Verification items for the finished model (mm, model axes). A direction names the side the tool comes from. Coordinates: 2 decimals unless noted, no trailing zeros. Order: outer loops, then holes, each group sorted by start corner. A loop starts at its lowest first (then second) coordinate and runs counter-clockwise, first axis right, second up. Notation, with made-up numbers: (82, -25) -> (97, -25) arc R24 cw to (97, 5) -> close; hole circle Ø6 at (13, 40.25). An arc over 180 degrees is marked (long way). Answer as CSV lines item,"result".
```python
from build123d import *

# Parameters (mm, degrees)
F0_W        = 10.5280357461
F0_H        = 21.2543252856
F1_DEPTH    = 30
F2_R        = 5
F3_R        = 2
F4_R        = 2
F5_R        = 2
F6_R        = 7
F7_T1_DEPTH = 81.4336597593
F8_R        = 10
F9_R        = 1
F10_R       = 10
F11_R       = 10
F13_DEPTH   = 30
F14_R       = 2


# Not quite as in the source:
# - a fillet or chamfer that OpenCascade refuses, or shapes differently, is made with other operations: its cross-section is extruded or revolved along the edge and cut away or added


with BuildPart() as f1:
    # F0 (on Top) → F1 (new body)
    with BuildSketch(Plane.XY):
        Polygon((23.4277165425, 17.0276444405), (-54.4175144403, 17.0276444405), (-54.4175144403, 8.6288927123), (12.8996807964, 8.6288927123), (23.4277165425, 8.6288927123), align=None)
        with Locations((18.1636986695, -1.9982699305)):
            Rectangle(F0_W, F0_H)
        Polygon((23.4277165425, -21.8901360014), (23.4277165425, -12.6254325733), (12.8996807964, -12.6254325733), (-40.6902853517, -12.6254325733), (-40.6902853517, -21.8901360014), (-27.7488247443, -21.8901360014), (-19.1767220313, -21.8901360014), align=None)
        with BuildLine():
            Line((-19.1767220313, -43.3673763092), (-19.1767220313, -21.8901360014))
            Line((-19.1767220313, -21.8901360014), (-27.7488247443, -21.8901360014))
            ThreePointArc((-27.7488247443, -21.8901360014), (-24.844212154, -33.1801228498), (-19.1767220313, -43.3673763092))
        make_face()
        with BuildLine():
            Line((-27.7488247443, -21.8901360014), (-40.6902853517, -21.8901360014))
            ThreePointArc((-40.6902853517, -21.8901360014), (-35.4626283769, -44.0139601174), (-20.8854291365, -61.4580781309))
            ThreePointArc((-20.8854291365, -61.4580781309), (-15.0806794225, -65.2011539101), (-8.8108392586, -68.098538912))
            ThreePointArc((-8.8108392586, -68.098538912), (11.6035028188, -71.235670703), (31.5175838768, -65.7569542527))
            Line((31.5175838768, -65.7569542527), (34.4113459094, -58.7176481952))
            ThreePointArc((34.4113459094, -58.7176481952), (5.0047282318, -60.1630877212), (-19.1767220313, -43.3673763092))
            ThreePointArc((-19.1767220313, -43.3673763092), (-24.844212154, -33.1801228498), (-27.7488247443, -21.8901360014))
        make_face()
        with BuildLine():
            ThreePointArc((-8.8108392586, -68.098538912), (-15.0806794225, -65.2011539101), (-20.8854291365, -61.4580781309))
            ThreePointArc((-20.8854291365, -61.4580781309), (-8.8309401238, -90.1622048174), (20.5386656224, -100.4900241667))
            Line((20.5386656224, -100.4900241667), (22.6970568086, -95.7385333169))
            ThreePointArc((22.6970568086, -95.7385333169), (0.4530333538, -89.3168234963), (-8.8108392586, -68.098538912))
        make_face()
    extrude(amount=F1_DEPTH)

    # F2
    f2_edges = [f1.edges().sort_by_distance(p)[0] for p in [
        (31.517584, -65.756954, 15),
    ]]
    fillet(f2_edges, radius=F2_R)

    # F3
    f3_edges = [f1.edges().sort_by_distance(p)[0] for p in [
        (34.411346, -58.717648, 15),
    ]]
    fillet(f3_edges, radius=F3_R)

    # F4
    f4_edges = [f1.edges().sort_by_distance(p)[0] for p in [
        (22.697057, -95.738533, 15),
    ]]
    fillet(f4_edges, radius=F4_R)

    # F5
    f5_edges = [f1.edges().sort_by_distance(p)[0] for p in [
        (20.538666, -100.490024, 15),
    ]]
    fillet(f5_edges, radius=F5_R)

    # F6
    f6_edges = [f1.edges().sort_by_distance(p)[0] for p in [
        (23.427717, -21.890136, 15),
        (23.427717, 17.027644, 15),
    ]]
    fillet(f6_edges, radius=F6_R)

    # F7: chamfer of 10 on 1 edges, made by hand

    # F7_s2 → F7_t1 (cut)
    with BuildSketch(Plane.XY.offset(-25.7168298797)):
        Polygon((-44.4175144403, 17.0276444405), (-54.4175144403, 7.0276444405), (-54.4175144403, 17.0276444405), align=None)
    extrude(amount=F7_T1_DEPTH, mode=Mode.SUBTRACT)

    # F8
    f8_edges = [f1.edges().sort_by_distance(p)[0] for p in [
        (-44.417514, 17.027644, 15),
    ]]
    fillet(f8_edges, radius=F8_R)

    # F9
    f9_edges = [f1.edges().sort_by_distance(p)[0] for p in [
        (-52.816266, 8.628893, 15),
        (-40.690285, -12.625433, 15),
    ]]
    fillet(f9_edges, radius=F9_R)

    # F10
    f10_edges = [f1.edges().sort_by_distance(p)[0] for p in [
        (-19.176722, -21.890136, 15),
    ]]
    fillet(f10_edges, radius=F10_R)

    # F11
    f11_edges = [f1.edges().sort_by_distance(p)[0] for p in [
        (-19.176722, -43.367376, 15),
    ]]
    fillet(f11_edges, radius=F11_R)

    # F12 (on face) → F13 (cut)
    with BuildSketch(Plane.XY.offset(30)):
        Polygon((-21.8362864107, -22.6786807179), (-36.1205674708, -22.6786807179), (-29.5046903193, -41.924867779), align=None)
    extrude(amount=-F13_DEPTH, mode=Mode.SUBTRACT)

    # F14
    f14_edges = [f1.edges().sort_by_distance(p)[0] for p in [
        (-21.836286, -22.678681, 15),
        (-36.120567, -22.678681, 15),
        (-29.50469, -41.924868, 15),
    ]]
    fillet(f14_edges, radius=F14_R)


solid = f1.part
```
Item 1: Release check for a two-part mould opening along X. For faces 1 (the cylindrical face through (-23.15, -23.53, 14.79)), 2 (the flat face through (23.428, -3, 15)), 3 (the cylindrical face through (-29.449, -38.173, 14.79)), 4 (the flat face through (12.9, -2, 15)) record: +X half, -X half, draft (parallel to the pull), parting line (faces both ways), or undercut.
Answer list:
face 1,"undercut"
face 2,"+X half"
face 3,"undercut"
face 4,"-X half"
Item 2: Depth check by flat-ended pin: pin 1 Ø5 at (y, z) = (-29, 21.5) entering from -X; pin 2 Ø6 at (y, z) = (-31, 22.5) entering from -X; pin 3 Ø10 at (y, z) = (-32.5, 18.5) entering from -X. Enter the tip coordinate at first touch or a pass-through.
Answer list:
pin 1,"x = -40.47"
pin 2,"x = -40.31"
pin 3,"x = -40.37"
Item 3: Thickness scan on line 1 (Y direction, x = -15.5, z = 10.25); line 2 (Y direction, x = -30, z = 6.25); line 3 (Y direction, x = 8, z = 8.25). Record the ranges inside material, lowest first.
Answer list:
line 1,"-81.84 to -47.75, -24.14 to -12.63, 8.63 to 17.03"
line 2,"-52.59 to -38.07, -22.68 to -12.63, 8.63 to 17.03"
line 3,"-99.42 to -94.01, -71.31 to -60.91, -21.89 to -12.63, 8.63 to 17.03"
Item 4: Section check C-C, the plane x = 7.5. Record the boundary of the cut face in (y, z).
Answer list:
outline,"(-99.29, 0) -> (-93.8, 0) -> (-93.8, 30) -> (-99.29, 30) -> close; (-71.3, 0) -> (-60.8, 0) -> (-60.8, 30) -> (-71.3, 30) -> close; (-21.89, 0) -> (-12.63, 0) -> (-12.63, 30) -> (-21.89, 30) -> close; (8.63, 0) -> (17.03, 0) -> (17.03, 30) -> (8.63, 30) -> close"
Item 5: Tool access check on faces 5 (the flat face through (-29, -22.679, 15)), 6 (the cylindrical face through (-35.605, -43.726, 14.79)), 7 (the cylindrical face through (-18.549, -43.338, 15.21)). Record the directions out of +Z, -Z, +X, -X, +Y, -Y that give a thin tool (end or side, any length) a straight path to the whole face; none if there is none.
Answer list:
face 5,"+Z, -Z"
face 6,"+Z, -Z, -X, -Y"
face 7,"+Z, -Z, +X"
Item 6: Section check D-D, the plane y = -53.5. Record the boundary of the cut face in (x, z), plus the area to 3 significant figures.
Answer list:
outline,"(-29.26, 0) -> (-8.86, 0) -> (-8.86, 30) -> (-29.26, 30) -> close"
area,"612 mm2"
Item 7: Section check A-A, the plane x = -1.5. Record the boundary of the cut face in (y, z), plus the area to 3 significant figures.
Answer list:
outline,"(-95.58, 0) -> (-87.42, 0) -> (-87.42, 30) -> (-95.58, 30) -> close; (-70.25, 0) -> (-57.75, 0) -> (-57.75, 30) -> (-70.25, 30) -> close; (-21.89, 0) -> (-12.63, 0) -> (-12.63, 30) -> (-21.89, 30) -> close; (8.63, 0) -> (17.03, 0) -> (17.03, 30) -> (8.63, 30) -> close"
area,"1,150 mm2"
